Here's how the part is built. I have some questions about the finished solid (model axes, mm). A direction names the side the tool comes from. Round coordinates to 2 decimals unless told otherwise and drop trailing zeros. Write each loop counter-clockwise with the first axis right and the second up, starting at its lowest first coordinate (ties: lowest second). Pieces come first, ordered by that corner, then holes. Notation, with made-up numbers: (-39.5, 40) - (-29.5, 40) arc R14 ccw to (-29.5, 61) - close; hole circle Ø3 at (43, 50.25). An arc over 180 degrees is marked (long way). Return JSON: item names as keys, results as strings. Group by question number.
```python
from build123d import *

# Parameters (mm, degrees)
SKETCH1_W           = 140
SKETCH1_H           = 18
BOSS_EXTRUDE1_DEPTH = 85
SKETCH3_R           = 8
CUT_EXTRUDE2_DEPTH  = 18
SKETCH5_W           = 140
SKETCH5_H           = 100
BOSS_EXTRUDE5_DEPTH = 12
SKETCH8_R           = 20
SKETCH8_R_2         = 9
SKETCH8_R_3         = 27.5
SKETCH8_R_4         = 15
BOSS_EXTRUDE6_DEPTH = 18
CUT_EXTRUDE3_DEPTH  = 12


with BuildPart() as part:
    # Sketch1 → Boss-Extrude1 (new body)
    with BuildSketch(Plane.XY):
        with Locations((70, 9)):
            Rectangle(SKETCH1_W, SKETCH1_H)
    extrude(amount=BOSS_EXTRUDE1_DEPTH)

    # Sketch3 → Cut-Extrude2 (cut)
    with BuildSketch(Plane(origin=(0, 18, 0), x_dir=(1, 0, 0), z_dir=(0, 1, 0))):
        with Locations(Location((35, -55, 0), (0, 0, 180))):
            Circle(SKETCH3_R)
        with Locations(Location((105, -55, 0), (0, 0, 180))):
            Circle(SKETCH3_R)
    extrude(amount=-CUT_EXTRUDE2_DEPTH, mode=Mode.SUBTRACT)

    # Sketch5 → Boss-Extrude5 (add)
    with BuildSketch(Plane(origin=(0, 0, 0), x_dir=(-1, 0, 0), z_dir=(0, 0, -1))):
        with Locations((-70, 50)):
            Rectangle(SKETCH5_W, SKETCH5_H)
    extrude(amount=BOSS_EXTRUDE5_DEPTH)

    # Sketch8 → Boss-Extrude6 (add, symmetric)
    # profile 1 of 2: a face of its own
    with BuildSketch(Plane.XY):
        with Locations(Location((20, 56, 0), (0, 0, 180))):
            Circle(SKETCH8_R)
        with Locations((20, 56)):
            Circle(SKETCH8_R_2, mode=Mode.SUBTRACT)
    # profile 2 of 2: a face of its own
    with BuildSketch(Plane.XY):
        with Locations((90, 100)):
            Circle(SKETCH8_R_3)
        with Locations((90, 100)):
            Circle(SKETCH8_R_4, mode=Mode.SUBTRACT)
    extrude(amount=BOSS_EXTRUDE6_DEPTH, both=True)

    # Sketch10 → Cut-Extrude3 (cut)
    with BuildSketch(Plane.XY):
        Polygon((117.5, 100), (140, 18), (140, 100), align=None)
        with BuildLine():
            ThreePointArc((20.315557315, 75.997510435), (44.612918998, 82.365712085), (62.5, 100))
            Line((62.5, 100), (0, 100))
            Line((0, 100), (0, 56))
            ThreePointArc((0, 56), (5.857864376, 70.142135624), (20, 76))
            ThreePointArc((20, 76), (20.157783568, 75.999377599), (20.315557315, 75.997510435))
        make_face()
    extrude(amount=-CUT_EXTRUDE3_DEPTH, mode=Mode.SUBTRACT)


solid = part.part
```
1) Will these pins go through, and if not, where does the flat tip stop? pin 1 Ø5 at (x, y) = (104.5, 19.5) entering from -Z; pin 2 Ø10 at (x, z) = (47, 11) entering from +Y; pin 3 Ø13 at (x, z) = (96, -3.5) entering from +Y.
2) Imagine slicing it at B-B (x = 35). Please give me the cut outline in (y, z).
3) I need wall thicknesses on line 1 along Z through (x, y) = (35, 7.5); line 2 along Y through (x, z) = (20, -14.55); line 3 along X through (y, z) = (99, 11). Which ranges of each line are inside material? Lowest first, please.
4) Imagine slicing it at A-A (z = 55). Please give me the cut outline in (x, y).
5) For faces 1 (the flat face through (69, 18, 42)), 2 (the flat face through (90, 100, -6)), 3 (the flat face through (90, 94, 0)), 4 (the cylindrical face through (24.153, 48.015, -14.958)), which set-ups out of +Z, -Z, +X, -X, +Y, -Y let a thin tool reach every point of the face, with its end or its side?
6) If we mould it in two halves opening along X, with no side actions, what happens to faces 5 (the flat face through (69, 9, 85)), 6 (the flat face through (0, 15, 26)), 7 (the cylindrical face through (97.37, 9.13, 57.4)), 8 (the cylindrical face through (24.153, 48.015, 8.874))? For each: released by +X, released by -X, zero draft, split by the parting line, or undercut.
7) Imagine slicing it at D-D (z = 75). Please give me the cut outline in (x, y), plus the area to 3 significant figures.
8) Imagine slicing it at C-C (y = 103). Please give me the cut outline in (x, z).
Results found:
{
 "1": {"pin 1": "stops at z = -12", "pin 2": "stops at y = 18", "pin 3": "stops at y = 127.5"},
 "2": {"outline": "(0, -12) - (42.77, -12) - (42.77, -18) - (69.23, -18) - (69.23, -12) - (78.19, -12) - (78.19, 0) - (69.23, 0) - (69.23, 18) - (42.77, 18) - (42.77, 0) - (18, 0) - (18, 47) - (0, 47) - close; (0, 63) - (18, 63) - (18, 85) - (0, 85) - close"},
 "3": {"line 1": "z = -12 to 47, 63 to 85", "line 2": "y = 36 to 47, 65 to 76", "line 3": "x = 62.52 to 75.03, 104.97 to 117.48"},
 "4": {"outline": "(0, 0) - (27, 0) - (27, 18) - (0, 18) - close; (43, 0) - (97, 0) - (97, 18) - (43, 18) - close; (113, 0) - (140, 0) - (140, 18) - (113, 18) - close"},
 "5": {"face 1": "+Z, +X, -X", "face 2": "+Z, -Z", "face 3": "+Z", "face 4": "-Z"},
 "6": {"face 5": "zero draft", "face 6": "released by -X", "face 7": "undercut", "face 8": "undercut"},
 "7": {"outline": "(0, 0) - (140, 0) - (140, 18) - (0, 18) - close", "area": "2,520 mm²"},
 "8": {"outline": "(62.66, -18) - (75.3, -18) - (75.3, 18) - (62.66, 18) - close; (104.7, -18) - (117.34, -18) - (117.34, 18) - (104.7, 18) - close"}
}
